Work out the finished part from the listing and answer in its coordinate system (mm). A direction names the side the tool comes from. Give positions to 0.01 mm unless a question says otherwise; leave off trailing zeros. Order: outer loops, then holes, each group sorted by start corner. A loop starts at its lowest first (then second) coordinate and runs counter-clockwise, first axis right, second up. Notation, with made-up numbers: (44, 60) - (59, 60) arc R20 ccw to (59, 76) - close; hole circle Ø5 at (68.5, -20). An arc over 180 degrees is marked (long way). Put each result on its own line as item: value.
```python
from build123d import *

# Parameters (mm, degrees)
ESQUISSE1_R             = 2.5
BOSS_EXTRU_1_DEPTH      = 10.5
ENL_V_START             = -6
ENL_V_MAT_EXTRU_2_DEPTH = 6
CONG_1_R                = 0.3


with BuildPart() as part:
    # Esquisse1 → Boss.-Extru.1 (new body)
    with BuildSketch(Plane.XY):
        with Locations(Location((0, 0, 0), (0, 0, 180))):
            Circle(ESQUISSE1_R)
    extrude(amount=BOSS_EXTRU_1_DEPTH)

    # Esquisse3 → Enlèv. mat.-Extru.2 (cut)
    with BuildSketch(Plane.XY.offset(10.5).offset(ENL_V_START)):
        with BuildLine():
            Line((1.5, 2), (1.5, -2))
            ThreePointArc((1.5, -2), (2.5, 0), (1.5, 2))
        make_face()
        with BuildLine():
            Line((-1.5, -2), (-1.5, 2))
            ThreePointArc((-1.5, 2), (-2.5, 0), (-1.5, -2))
        make_face()
    extrude(amount=ENL_V_MAT_EXTRU_2_DEPTH, mode=Mode.SUBTRACT)

    # Congé1
    cong_1_edges = [part.edges().sort_by_distance(p)[0] for p in [
        (0, 2.5, 10.5),
        (0, -2.5, 10.5),
    ]]
    fillet(cong_1_edges, radius=CONG_1_R)


solid = part.part
```
(1) Section A-A, the plane y = 0 is taken. Write down the section's boundary in (x, z), then the cut area to 3 significant figures.
Geometry check:
outline: (-2.5, 0) - (2.5, 0) - (2.5, 4.5) - (1.5, 4.5) - (1.5, 10.5) - (-1.5, 10.5) - (-1.5, 4.5) - (-2.5, 4.5) - close
area: 40.5 mm²
(2) Section C-C, the plane x = -2.05 is taken. Write down the section's boundary in (y, z), then the cut area to 3 significant figures.
Geometry check:
outline: (-1.43, 0) - (1.43, 0) - (1.43, 4.5) - (-1.43, 4.5) - close
area: 12.9 mm²
(3) Section B-B, the plane z = 6 is taken. Write down the section's boundary in (x, y).
Geometry check:
outline: (-1.5, -2) arc R2.5 ccw to (1.5, -2) - (1.5, 2) arc R2.5 ccw to (-1.5, 2) - close
(4) Section D-D, the plane y = 1.45 is taken. Write down the section's boundary in (x, z).
Geometry check:
outline: (-2.04, 0) - (2.04, 0) - (2.04, 4.5) - (1.5, 4.5) - (1.5, 10.5) - (-1.5, 10.5) - (-1.5, 4.5) - (-2.04, 4.5) - close
(5) Given pin 1 (0.8 mm diameter, centred on x = 2, y = -1, fed in from +Z); pin 2 (3 mm diameter, centred on y = 0.5, z = 8, fed in from +X), each flat-ended and moving along its own axis, determine where each tip first touches the part or whether it passes through.
Geometry check:
pin 1: stops at z = 4.5
pin 2: stops at x = 1.5
(6) A tool of negligible diameter and unlimited length cuts with its end or side. For faces 1 (the face through (0, 0, 0)), 2 (the face through (2, 0, 4.5)), 3 (the face through (-2, 0, 4.5)), from which of +Z, -Z, +X, -X, +Y, -Y can it reach the whole face along a straight path? Write none if from no direction.
Geometry check:
face 1: -Z, +X, -X, +Y, -Y
face 2: +Z, +X, +Y, -Y
face 3: +Z, -X, +Y, -Y
(7) Straight lines are drawn through the part: line 1 (X direction, y = 1.05, z = 7.5); line 2 (Z direction, x = 2.05, y = 0.05); line 3 (X direction, y = -1.9, z = 3.25). For each, find the intervals that lie inside material, in ascending order.
Geometry check:
line 1: x = -1.5 to 1.5
line 2: z = 0 to 4.5
line 3: x = -1.62 to 1.62
